from build123d import *

# Parameters (mm, degrees)
F1_DEPTH = 5.5
F2_R     = 4
F3_DEPTH = 75
F6_SIZE  = 0.7


with BuildPart() as f1:
    # F0 (on Top) → F1 (new body)
    with BuildSketch(Plane.XY):
        Polygon((0, -7.505553), (6.5, -3.752777), (6.5, 3.752777), (0, 7.505553), (-6.5, 3.752777), (-6.5, -3.752777), align=None)
    extrude(amount=F1_DEPTH)

    # F2 (on face) → F3 (join)
    with BuildSketch(Plane.XY.offset(5.5)):
        Circle(F2_R)
    extrude(amount=F3_DEPTH)

    # F4 (on Front) → F5 (revolve, cut)
    with BuildSketch(Plane.XZ):
        Polygon((11.157986, 2.68929), (6.5, 0), (11.157986, 0), align=None)
    revolve(axis=Axis((0, 0, 4.89242), (0, 0, 1)), mode=Mode.SUBTRACT)

    # F6
    f6_edges = [f1.edges().sort_by_distance(p)[0] for p in [
        (-4, 0, 80.5),
    ]]
    chamfer(f6_edges, length=F6_SIZE)


solid = f1.part
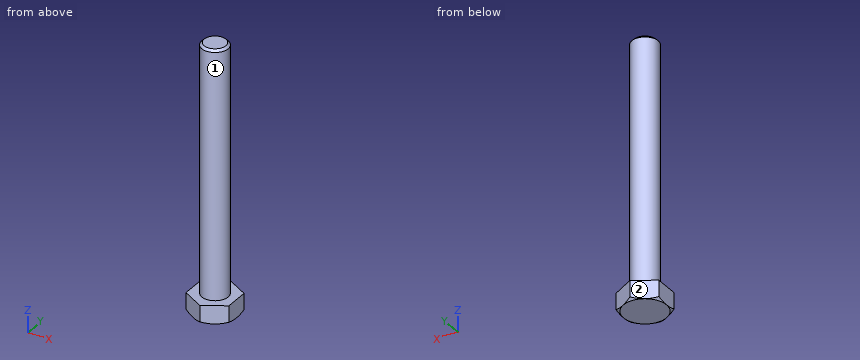
Can you work these out from the model? Positions are in its coordinate system, mm. Face numbers are marked on the shaded views. A direction names the side the tool comes from. Coordinates: 2 decimals unless noted, no trailing zeros. Write each loop counter-clockwise with the first axis right and the second up, starting at its lowest first coordinate (ties: lowest second). Pieces come first, ordered by that corner, then holes. Notation, with made-up numbers: (-32, 48.25) -> (-22, 48.25) arc R15 ccw to (-22, 76.25) -> close; hole circle Ø4 at (-13.75, 40). An arc over 180 degrees is marked (long way). Write each question's results on one line, items separated by ' | '. Start each with the question number.
Item 1: If we section it at A-A, the plane z = 15.5: Write out the boundary of the cut face in (x, y).
Item 2: On a 3-axis mill with a long thin cutter (end or side, diameter ignored), from which of +Z, -Z, +X, -X, +Y, -Y can I reach the whole of each face in a straight line? I mean the marked faces 1 and 2. Say none if no direction works.
Item 3: Please list where these lines run through material, in increasing order: probe 1 along Z at (x, y) = (-4.5, 2.25); probe 2 along Y at (x, z) = (0, 24); probe 3 along Y at (x, z) = (-2.25, 37.5).
Item 4: I'm going to push flat-ended pins straight in: P1, Ø3, axis at x = -4, y = 4.5, coming from the -Z side; P2, Ø4, axis at x = 1, z = 52, coming from the +Y side; P3, Ø2, axis at y = 2.5, z = 59.5, coming from the -X side; P4, Ø3, axis at x = 3, z = 31.5, coming from the +Y side. Where does each tip first touch, or does it pass through?
Answer block:
1) outline: circle Ø8 at (0, 0)
2) face 1: +Z | face 2: +Z, -Z, -X, +Y
3) probe 1: 0 to 5.5 | probe 2: -4 to 4 | probe 3: -3.31 to 3.31
4) P1: z = 0 | P2: y = 4 | P3: x = -3.71 | P4: y = 3.71
